from build123d import *

# Parameters (mm, degrees)
EXTRUDE_3_DEPTH     = 4
FILLET_3_R          = 20
FILLET_4_R          = 20
FILLET_5_R          = 20
FILLET_6_R          = 20
FILLET_7_R          = 20
FILLET_8_R          = 20
FILLET_9_R          = 20
FILLET_10_R         = 20
SKETCH_6_R          = 1.75
CUT_EXTRUDE_3_DEPTH = 4
SKETCH_7_R          = 2
CUT_EXTRUDE_4_DEPTH = 4


with BuildPart() as part:
    # Эскиз5 → Бобышка-Вытянуть3 (new body)
    with BuildSketch(Plane(origin=(0, 0, 0), x_dir=(1, 0, 0), z_dir=(0, 1, 0))):
        with BuildLine():
            Line((-100, 130), (-74.963405707, 109.970724565))
            ThreePointArc((-74.963405707, 109.970724565), (0, 83.674981698), (74.963405707, 109.970724565))
            Line((74.963405707, 109.970724565), (100, 130))
            ThreePointArc((100, 130), (122.809833424, 122.809833424), (130, 100))
            Line((130, 100), (109.970724565, 74.963405707))
            ThreePointArc((109.970724565, 74.963405707), (83.674981698, 0), (109.970724565, -74.963405707))
            Line((109.970724565, -74.963405707), (130, -100))
            ThreePointArc((130, -100), (122.809833424, -122.809833424), (100, -130))
            Line((100, -130), (74.963405707, -109.970724565))
            ThreePointArc((74.963405707, -109.970724565), (0, -83.674981698), (-74.963405707, -109.970724565))
            Line((-74.963405707, -109.970724565), (-100, -130))
            ThreePointArc((-100, -130), (-122.809833424, -122.809833424), (-130, -100))
            Line((-130, -100), (-109.970724565, -74.963405707))
            ThreePointArc((-109.970724565, -74.963405707), (-83.674981698, 0), (-109.970724565, 74.963405707))
            Line((-109.970724565, 74.963405707), (-130, 100))
            ThreePointArc((-130, 100), (-122.809833424, 122.809833424), (-100, 130))
        make_face()
    extrude(amount=EXTRUDE_3_DEPTH)

    # Скругление3
    fillet_3_edges = [part.edges().sort_by_distance(p)[0] for p in [
        (130, 2, -100),
    ]]
    fillet(fillet_3_edges, radius=FILLET_3_R)

    # Скругление4
    fillet_4_edges = [part.edges().sort_by_distance(p)[0] for p in [
        (100, 2, -130),
    ]]
    fillet(fillet_4_edges, radius=FILLET_4_R)

    # Скругление5
    fillet_5_edges = [part.edges().sort_by_distance(p)[0] for p in [
        (-100, 2, -130),
    ]]
    fillet(fillet_5_edges, radius=FILLET_5_R)

    # Скругление6
    fillet_6_edges = [part.edges().sort_by_distance(p)[0] for p in [
        (-130, 2, -100),
    ]]
    fillet(fillet_6_edges, radius=FILLET_6_R)

    # Скругление7
    fillet_7_edges = [part.edges().sort_by_distance(p)[0] for p in [
        (-100, 2, 130),
    ]]
    fillet(fillet_7_edges, radius=FILLET_7_R)

    # Скругление8
    fillet_8_edges = [part.edges().sort_by_distance(p)[0] for p in [
        (-130, 2, 100),
    ]]
    fillet(fillet_8_edges, radius=FILLET_8_R)

    # Скругление9
    fillet_9_edges = [part.edges().sort_by_distance(p)[0] for p in [
        (100, 2, 130),
    ]]
    fillet(fillet_9_edges, radius=FILLET_9_R)

    # Скругление10
    fillet_10_edges = [part.edges().sort_by_distance(p)[0] for p in [
        (130, 2, 100),
    ]]
    fillet(fillet_10_edges, radius=FILLET_10_R)

    # Эскиз6 → Вырез-Вытянуть3 (cut)
    with BuildSketch(Plane(origin=(0, 4, 0), x_dir=(1, 0, 0), z_dir=(0, 1, 0))):
        with Locations(Location((-104.5, 104.5, 0), (0, 0, 270))):
            Circle(SKETCH_6_R)
        with Locations(Location((104.5, 104.5, 0), (0, 0, 270))):
            Circle(SKETCH_6_R)
        with Locations(Location((104.5, -104.5, 0), (0, 0, 270))):
            Circle(SKETCH_6_R)
        with Locations(Location((-104.5, -104.5, 0), (0, 0, 270))):
            Circle(SKETCH_6_R)
    extrude(amount=-CUT_EXTRUDE_3_DEPTH, mode=Mode.SUBTRACT)

    # Эскиз7 → Вырез-Вытянуть4 (cut)
    with BuildSketch(Plane(origin=(0, 4, 0), x_dir=(1, 0, 0), z_dir=(0, 1, 0))):
        with Locations(Location((-40, 40, 0), (0, 0, 270))):
            Circle(SKETCH_7_R)
        with Locations(Location((40, 40, 0), (0, 0, 270))):
            Circle(SKETCH_7_R)
        with Locations(Location((40, -40, 0), (0, 0, 270))):
            Circle(SKETCH_7_R)
        with Locations(Location((-40, -40, 0), (0, 0, 270))):
            Circle(SKETCH_7_R)
    extrude(amount=-CUT_EXTRUDE_4_DEPTH, mode=Mode.SUBTRACT)


solid = part.part
CAD build for the part. Positions are in the model's coordinates, mm. A direction names the side the tool comes from. Give positions to 0.01 mm unless a question says otherwise; leave off trailing zeros. Write each loop counter-clockwise with the first axis right and the second up, starting at its lowest first coordinate (ties: lowest second). Pieces come first, ordered by that corner, then holes. Notation, with made-up numbers: (65, 58.5) - (122, 58.5) arc R29 ccw to (122, 84.5) - close; hole circle Ø7 at (2, 83). An arc over 180 degrees is marked (long way). Put each result on its own line as item: value.
(1) Saw through at B-B (z = 91). List the corners of the cut face in (x, y), then the cut area to 3 significant figures.
Working result:
outline: (-122.8, 0) - (-41.28, 0) - (-41.28, 4) - (-122.8, 4) - close; (41.28, 0) - (122.8, 0) - (122.8, 4) - (41.28, 4) - close
area: 652 mm^2
(2) Saw through at D-D (z = 12.5). List the corners of the cut face in (x, y), then the cut area to 3 significant figures.
Working result:
outline: (-84.33, 0) - (84.33, 0) - (84.33, 4) - (-84.33, 4) - close
area: 675 mm^2
(3) Pull direction X, two halves, no side cores. Call faces 1 (the flat face through (85, 2, -118)), 2 (the flat face through (-118, 2, 85)), 3 (the flat face through (2, 4, -2)): released by +X, released by -X, zero draft, split by the parting line, or undercut.
Working result:
face 1: undercut
face 2: released by -X
face 3: zero draft
(4) Drop flat-ended pins along their axis: pin 1 Ø3 at (x, z) = (-40, 40) entering from +Y; pin 2 Ø5.5 at (x, z) = (-104.5, -104.5) entering from +Y; pin 3 Ø1 at (x, y) = (31, 3.5) entering from +Z. Give the stop position or say it passes through.
Working result:
pin 1: through
pin 2: y = 4
pin 3: z = 87.88
(5) Tool access for faces 4 (the flat face through (-118, 2, -85)), 5 (the flat face through (-85, 2, -118)), 6 (the flat face through (85, 2, 118)), 7 (the flat face through (118, 2, 85)), 8 (the cylindrical face through (122.904, 1.972, 122.715)): list every direction of +Z, -Z, +X, -X, +Y, -Y with a clear straight run to the whole face (end or side of a thin tool).
Working result:
face 4: -X, +Y, -Y
face 5: -Z, +Y, -Y
face 6: +Z, +Y, -Y
face 7: +X, +Y, -Y
face 8: +Z, +X, +Y, -Y
(6) Wall check: L1, parallel to Z at x = -104.5, y = 1.25; L2, parallel to X at y = 1.9, z = 40. Give the ranges that are in metal, low to high.
Working result:
L1: -129.75 to -106.25, -102.75 to -67.56, 67.56 to 102.75, 106.25 to 129.75
L2: -90.54 to -42, -38 to 38, 42 to 90.54
(7) Saw through at C-C (z = -99.5). List the corners of the cut face in (x, y).
Working result:
outline: (-128.48, 0) - (-59.56, 0) - (-59.56, 4) - (-128.48, 4) - close; (59.56, 0) - (128.48, 0) - (128.48, 4) - (59.56, 4) - close
(8) Saw through at A-A (y = 2.6). Count the separate pieces of the cut face and the enclosed holes in it, then the cut area to 3 significant figures.
Working result:
separate pieces: 1
enclosed holes: 8
area: 42,200 mm^2
